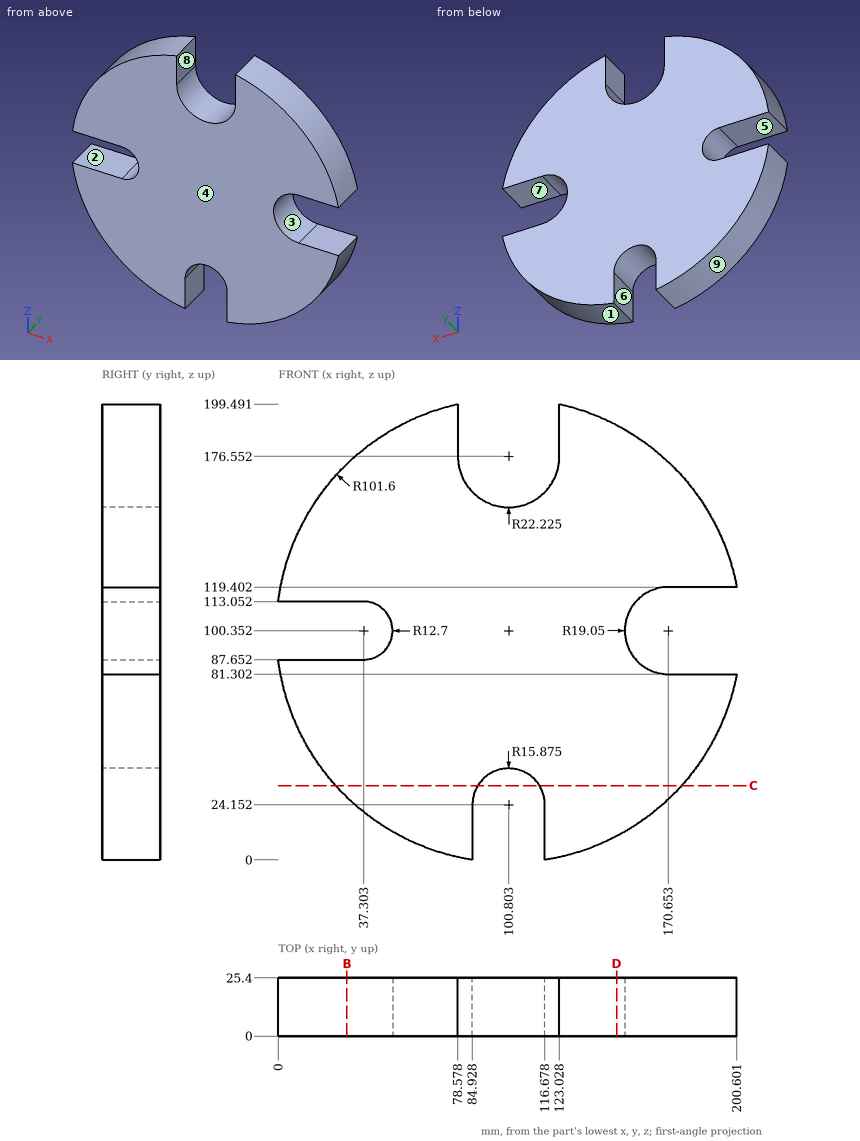
For this review, use the dimensioned drawing (mm, ordinates from the lowest corner) and the shaded views. A direction names the side the tool comes from. Give positions to 0.01 mm unless a question says otherwise; leave off trailing zeros. Loops run counter-clockwise (first coordinate to the right, second up) from the corner with the lowest first, then second, coordinate; pieces in that order, holes last.
Item 1: Draft analysis for pull direction Z (two halves, no side actions). For the marked faces 1, 2, 3 and 4, state which applies: +Z half, -Z half, draft (parallel to the pull), parting line (faces both ways), or undercut.
Item 2: Tool access review of the marked faces 5, 6, 7, 8 and 9: name each direction out of +Z, -Z, +X, -X, +Y, -Y from which nothing blocks a thin tool from reaching the whole face with its end or side.
Item 3: Take a section at B-B, the plane x = 30. State the section outline as (y, z) points.
Item 4: For line 1 along X through (y, z) = (6.25, 161) (1 decimal); line 2 along Z through (x, y) = (102, 13); line 3 along Z through (x, y) = (175.5, 7.5) (1 decimal), list the stretches that pass through material, from the lowest coordinate up.
Item 5: Insertion check: pin 1 (5 mm diameter, centred on y = 9.5, z = 121.5, fed in from -X); pin 2 (8 mm diameter, centred on x = 180, z = 164.5, fed in from -Y); pin 3 (10 mm diameter, centred on y = 10, z = 48.5, fed in from -X); pin 4 (7.5 mm diameter, centred on x = 181.5, y = 6.5, fed in from -Z) (1 decimal). Each pin has a flat end and moves straight along its axis. Give the tip position at first contact, or say it passes through.
Item 6: Take a section at D-D, the plane x = 148. State the section outline as (y, z) points (1 decimal).
Item 7: Take a section at C-C, the plane z = 32.5. State the section outline as (x, y) points (1 decimal), and give its area (3 significant figures).
Calculated:
1. face 1: -Z half
1. face 2: undercut
1. face 3: undercut
1. face 4: draft
2. face 5: -X, +Y, -Y
2. face 6: -Z, +Y, -Y
2. face 7: +X, +Y, -Y
2. face 8: +Z, +Y, -Y
2. face 9: -Z, -X, +Y, -Y
3. outline: (0, 27.49) - (25.4, 27.49) - (25.4, 87.65) - (0, 87.65) - close; (0, 113.05) - (25.4, 113.05) - (25.4, 173.22) - (0, 173.22) - close
4. line 1: x = 19.3 to 84.9, 116.7 to 182.3
4. line 2: z = 39.98 to 154.36
4. line 3: z = 31.5 to 81.3, 119.4 to 169.2
5. pin 1: stops at x = 0.93
5. pin 2: stops at y = 0
5. pin 3: stops at x = 10.65
5. pin 4: stops at z = 34
6. outline: (0, 10.4) - (25.4, 10.4) - (25.4, 190.3) - (0, 190.3) - close
7. outline: (25.2, 0) - (87.3, 0) - (87.3, 25.4) - (25.2, 25.4) - close; (114.3, 0) - (176.4, 0) - (176.4, 25.4) - (114.3, 25.4) - close
7. area: 3,160 mm2
